Input: dimensioned drawing with shaded views. Units: mm. Origin: part minimum x, y, z. Round coordinates to 2 decimals unless told otherwise and drop trailing zeros. Loops run counter-clockwise (first coordinate to the right, second up) from the corner with the lowest first, then second, coordinate; pieces in that order, holes last. Notation, with made-up numbers: M 62.25,-24 L 112.25,-24 A21 ccw 112.25,-3 Z; hole C 49.25,71.5 d10. An arc over 180 degrees is marked long. One line per item, written item: value.
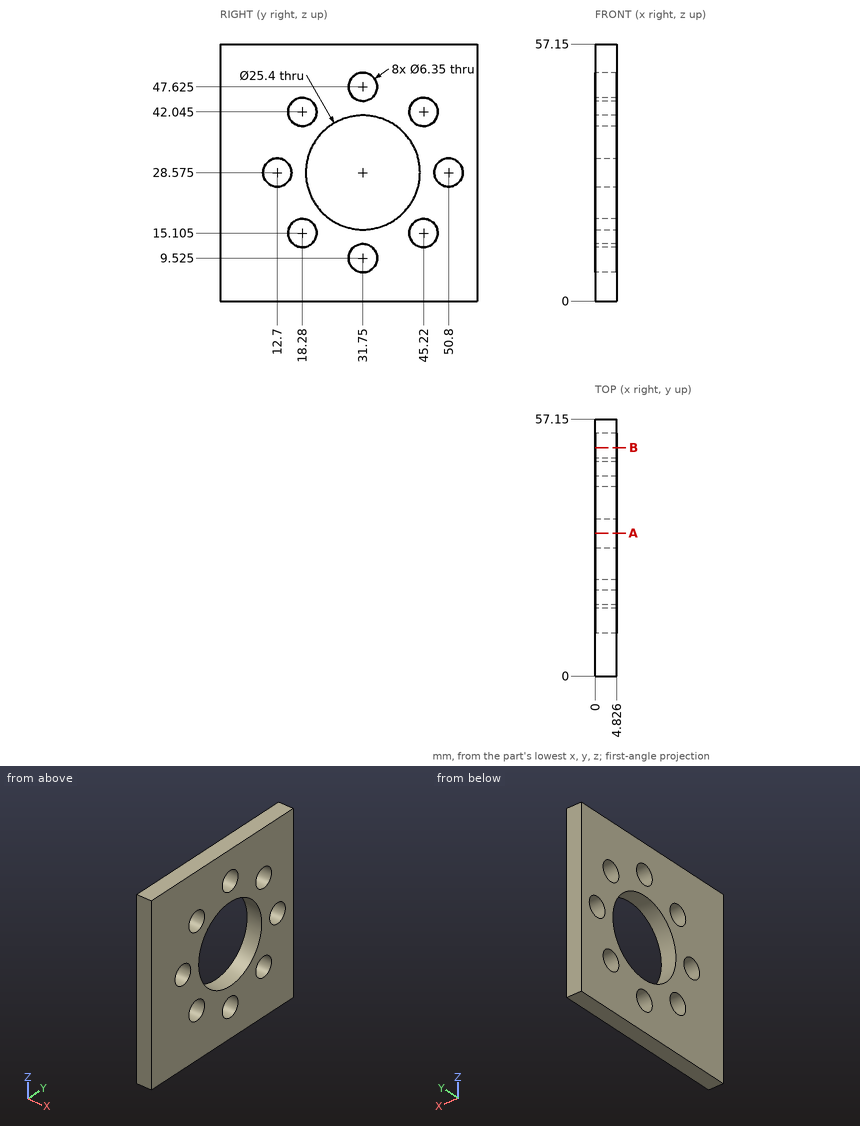
1. Ray query, line 1 (Y direction, x = 1.25, z = 15); line 2 (Y direction, x = 2.8, z = 29.5); line 3 (Y direction, x = 1, z = 20.5). Return the intervals inside material, ascending. Write a range as [from, to].
Report:
line 1: y = [0, 15.11], [21.45, 42.05], [48.39, 57.15]
line 2: y = [0, 9.66], [15.74, 19.08], [44.42, 47.76], [53.84, 57.15]
line 3: y = [0, 21.95], [41.55, 57.15]
2. Section query A-A (y = 31.75). Count the separate pieces of the cut face and the enclosed holes in it.
Report:
separate pieces: 4
enclosed holes: 0
3. Section query B-B (y = 50.8). Return the cut outline in (x, z), and give its area (3 significant figures).
Report:
outline: M 0,0 L 4.83,0 L 4.83,25.4 L 0,25.4 Z; M 0,31.75 L 4.83,31.75 L 4.83,57.15 L 0,57.15 Z
area: 245 mm2
